```python
from build123d import *

# Parameters (mm, degrees)
BOSS_EXTRUDE1_DEPTH = 5.35


with BuildPart() as part:
    # Model → Boss-Extrude1 (new body)
    with BuildSketch(Plane.XY):
        with BuildLine():
            Line((59.055, 31.35), (70, 31.35))
            Line((70, 31.35), (70, 18.35))
            Line((70, 18.35), (65, 18.35))
            Line((65, 18.35), (65, 13))
            Line((65, 13), (70, 13))
            Line((70, 13), (70, 0))
            Line((70, 0), (64, 0))
            Line((64, 0), (64, 5.35))
            Line((64, 5.35), (6, 5.35))
            Line((6, 5.35), (6, 0))
            Line((6, 0), (0, 0))
            Line((0, 0), (0, 13))
            Line((0, 13), (5, 13))
            Line((5, 13), (5, 18.35))
            Line((5, 18.35), (0, 18.35))
            Line((0, 18.35), (0, 31.35))
            Line((0, 31.35), (10.945, 31.35))
            ThreePointArc((10.945, 31.35), (35, 7.295), (59.055, 31.35))
        make_face()
    extrude(amount=BOSS_EXTRUDE1_DEPTH)


solid = part.part
```
Design review of the part built by this model. Coordinates are the model's own, in mm. A direction names the side the tool comes from. Round coordinates to 2 decimals unless told otherwise and drop trailing zeros. Order: outer loops, then holes, each group sorted by start corner. A loop starts at its lowest first (then second) coordinate and runs counter-clockwise, first axis right, second up. Notation, with made-up numbers: M 2,-14.5 L 9,-14.5 A21 ccw 9,-8.5 Z; hole C 39.5,11 d7. An arc over 180 degrees is marked long. Put each result on its own line as item: value.
Q1. Consider section D-D (y = 10). State the section outline as (x, z) points, and give its area (3 significant figures).
Reported:
outline: M 0,0 L 23.92,0 L 23.92,5.35 L 0,5.35 Z; M 46.08,0 L 70,0 L 70,5.35 L 46.08,5.35 Z
area: 256 mm²
Q2. To check wall thickness, follow line 1 (Y direction, x = 66.5, z = 0.6); line 2 (X direction, y = 4, z = 2.95); line 3 (Y direction, x = 34.5, z = 2.5). State the ranges of each line that lie inside material, in increasing order.
Reported:
line 1: 0 to 13, 18.35 to 31.35
line 2: 0 to 6, 64 to 70
line 3: 5.35 to 7.3
Q3. Consider section C-C (x = 35). State the section outline as (y, z) points (3 decimals).
Reported:
outline: M 5.35,0 L 7.295,0 L 7.295,5.35 L 5.35,5.35 Z
Q4. Consider section A-A (z = 4.1). State the section outline as (x, y) points (3 decimals).
Reported:
outline: M 0,0 L 6,0 L 6,5.35 L 64,5.35 L 64,0 L 70,0 L 70,13 L 65,13 L 65,18.35 L 70,18.35 L 70,31.35 L 59.055,31.35 A24.055 cw 10.945,31.35 L 0,31.35 L 0,18.35 L 5,18.35 L 5,13 L 0,13 Z
Q5. Machinability: for faces 1 (the face through (5, 31.35, 3)), 2 (the face through (67, 13, 3)), 3 (the face through (35, 5.35, 3)), 4 (the face through (2, 13, 3)), which of the approach directions +Z, -Z, +X, -X, +Y, -Y give a long, thin tool a straight path to every point of the face, cutting with its end or side? Answer none if there is none.
Reported:
face 1: +Z, -Z, +X, -X, +Y
face 2: +Z, -Z, +X
face 3: +Z, -Z, -Y
face 4: +Z, -Z, -X
Q6. Insertion check: pin 1 Ø1.6 at (x, z) = (45.5, 4) entering from -Y; pin 2 Ø3 at (x, z) = (39.5, 4.5) entering from +Y; pin 3 Ø1.5 at (y, z) = (15.5, 3.5) entering from -X. Each pin has a flat end and moves straight along its axis. Give the tip position at first contact, or say it passes through.
Reported:
pin 1: y = 5.35
pin 2: y = 8.06
pin 3: x = 5
Q7. Consider section B-B (y = 15). State the section outline as (x, z) points.
Reported:
outline: M 5,0 L 17.36,0 L 17.36,5.35 L 5,5.35 Z; M 52.64,0 L 65,0 L 65,5.35 L 52.64,5.35 Z
